Check sheet for the modelled part. Datum: model origin and axes. Units: mm. Face numbers are marked on the shaded views. A direction names the side the tool comes from. Round coordinates to 2 decimals unless told otherwise and drop trailing zeros. Order: outer loops, then holes, each group sorted by start corner. A loop starts at its lowest first (then second) coordinate and runs counter-clockwise, first axis right, second up. Notation, with made-up numbers: (62.25, 4.25) -> (83.25, 4.25) arc R10 cw to (83.25, 13.25) -> close; hole circle Ø4 at (28.5, -4.5). An arc over 180 degrees is marked (long way). Use CSV: the item, a comma, the result in double quotes.
```python
from build123d import *

# Parameters (mm, degrees)
SKETCH2_W          = 3
SKETCH2_H          = 6
CUT_EXTRUDE1_DEPTH = 56.009090158
CHAMFER1_SIZE      = 0.5


with BuildPart() as part:
    # Sketch1 → Revolve1 (revolve)
    with BuildSketch(Plane(origin=(0, 0, 0), x_dir=(1, 0, 0), z_dir=(0, 1, 0))):
        Polygon((-4, 25.890517241), (-35, 25.890517241), (-35, 25.290517241), (-34.5, 25.290517241), (-34.5, 18.090517241), (-35, 18.090517241), (-35, 17.490517241), (-34.5, 17.490517241), (-34.5, 10.290517241), (-35, 10.290517241), (-35, 9.690517241), (-34.5, 9.690517241), (-34.5, 2.490517241), (-35, 2.490517241), (-35, 1.890517241), (-4, 1.890517241), align=None)
    revolve(axis=Axis((0, 0, -42.552298851), (0, 0, 1)))

    # Sketch2 → Cut-Extrude1 (cut, through all)
    with BuildSketch(Plane(origin=(0, 0, -25.890517241), x_dir=(-1, 0, 0), z_dir=(0, 0, -1))):
        with Locations((0, 3)):
            Rectangle(SKETCH2_W, SKETCH2_H)
    extrude(amount=-CUT_EXTRUDE1_DEPTH, mode=Mode.SUBTRACT)

    # Chamfer1
    chamfer1_edges = [part.edges().sort_by_distance(p)[0] for p in [
        (0, -4, -25.890517241),
        (-1.5, 4.854049622, -25.890517241),
        (0, -4, -1.890517241),
        (-1.5, 4.854049622, -1.890517241),
        (1.5, 4.854049622, -1.890517241),
        (0, 6, -1.890517241),
        (0, 6, -25.890517241),
        (1.5, 4.854049622, -25.890517241),
    ]]
    chamfer(chamfer1_edges, length=CHAMFER1_SIZE)


solid = part.part
```
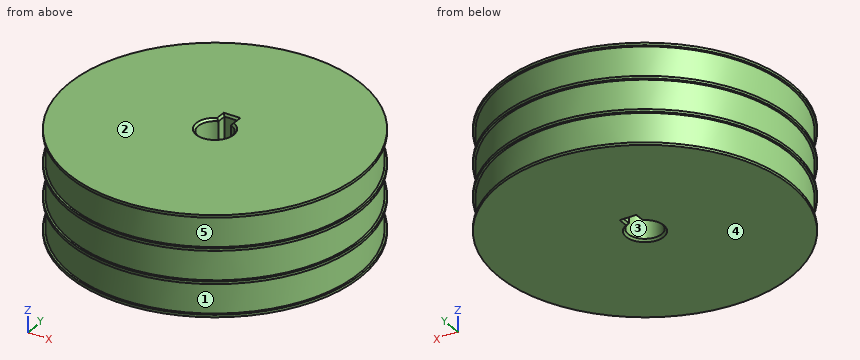
Q1. Scan lines: L1, parallel to X at y = 0, z = -11.5; L2, parallel to Y at x = 0, z = -8.5; L3, parallel to Y at x = 0, z = -10.25. Record each from-to range of solid material in increasing order.
Result sheet:
L1,"x = -34.5 to -4, 4 to 34.5"
L2,"y = -34.5 to -4, 6 to 34.5"
L3,"y = -35 to -4, 6 to 35"
Q2. Sectioned sample at A-A, the plane z = -5. Enter the section's corners in (x, y), then the cut area to 3 significant figures.
Result sheet:
outline,"circle Ø69 at (0, 0); hole (-1.5, 3.71) arc R4 ccw (long way) to (1.5, 3.71) -> (1.5, 6) -> (-1.5, 6) -> close"
area,"3,680 mm^2"
Q3. Sectioned sample at C-C, the plane y = 23. Enter the section's corners in (x, z).
Result sheet:
outline,"(-26.38, -25.89) -> (26.38, -25.89) -> (26.38, -25.29) -> (25.71, -25.29) -> (25.71, -18.09) -> (26.38, -18.09) -> (26.38, -17.49) -> (25.71, -17.49) -> (25.71, -10.29) -> (26.38, -10.29) -> (26.38, -9.69) -> (25.71, -9.69) -> (25.71, -2.49) -> (26.38, -2.49) -> (26.38, -1.89) -> (-26.38, -1.89) -> (-26.38, -2.49) -> (-25.71, -2.49) -> (-25.71, -9.69) -> (-26.38, -9.69) -> (-26.38, -10.29) -> (-25.71, -10.29) -> (-25.71, -17.49) -> (-26.38, -17.49) -> (-26.38, -18.09) -> (-25.71, -18.09) -> (-25.71, -25.29) -> (-26.38, -25.29) -> close"
Q4. Access from +Z, -Z, +X, -X, +Y, -Y to the whole of each face (thin tool, end or side, straight path). Record for the marked faces 4 and 5.
Result sheet:
face 4,"-Z, +X, -X, +Y, -Y"
face 5,"none"
Q5. Go/stop test with flat-tipped pins: pin 1 (8 mm diameter, centred on y = -8, z = -19.5, fed in from +X); pin 2 (10 mm diameter, centred on y = -16, z = -14, fed in from -X); pin 3 (2.5 mm diameter, centred on x = 0.5, z = -16.5, fed in from -Y). Record where each tip stops, or that it passes through.
Result sheet:
pin 1,"stops at x = 34.74"
pin 2,"stops at x = -32.72"
pin 3,"stops at y = -35"
Q6. Sectioned sample at B-B, the plane x = 14. Enter the section's corners in (y, z).
Result sheet:
outline,"(-32.08, -25.89) -> (32.08, -25.89) -> (32.08, -25.29) -> (31.53, -25.29) -> (31.53, -18.09) -> (32.08, -18.09) -> (32.08, -17.49) -> (31.53, -17.49) -> (31.53, -10.29) -> (32.08, -10.29) -> (32.08, -9.69) -> (31.53, -9.69) -> (31.53, -2.49) -> (32.08, -2.49) -> (32.08, -1.89) -> (-32.08, -1.89) -> (-32.08, -2.49) -> (-31.53, -2.49) -> (-31.53, -9.69) -> (-32.08, -9.69) -> (-32.08, -10.29) -> (-31.53, -10.29) -> (-31.53, -17.49) -> (-32.08, -17.49) -> (-32.08, -18.09) -> (-31.53, -18.09) -> (-31.53, -25.29) -> (-32.08, -25.29) -> close"
Q7. Mould release check, pull along Z, two halves, no side actions. Record for the marked faces 1, 2 and 3: pulls with the +Z half, pulls with the -Z half, needs draft (parallel to the pull), parting line crosses it, or undercut.
Result sheet:
face 1,"undercut"
face 2,"pulls with the +Z half"
face 3,"needs draft"
